from build123d import *

# Parameters (mm, degrees)
SKETCH_W        = 60
SKETCH_H        = 10
PAD_DEPTH       = 3
SKETCH001_R     = 2
POCKET_DEPTH    = 124.80412
SKETCH002_R     = 2.5
PAD001_DEPTH    = 40
FILLET_R        = 2
SKETCH003_W     = 12
SKETCH003_H     = 5
PAD002_DEPTH    = 5
SKETCH004_W     = 8
SKETCH004_H     = 3
POCKET001_DEPTH = 7.501
FILLET001_R     = 2
FILLET002_R     = 3


with BuildPart() as part:
    # Sketch → Pad (new body)
    with BuildSketch(Plane.XY):
        Rectangle(SKETCH_W, SKETCH_H)
    extrude(amount=PAD_DEPTH)

    # Sketch001 (on Face6 of Pad) → Pocket (cut, through all)
    with BuildSketch(Plane.XY.offset(3)):
        with Locations((-20, 0)):
            Circle(SKETCH001_R)
    pocket = extrude(amount=-POCKET_DEPTH, mode=Mode.SUBTRACT)

    # Mirrored: Pocket across Sketch001 V_Axis
    add(pocket.mirror(Plane(origin=(0, 0, 3), x_dir=(0, 0, 1), z_dir=(1, 0, 0))), mode=Mode.SUBTRACT)

    # Sketch002 (on Face5 of Mirrored) → Pad001 (join)
    with BuildSketch(Plane.XY.offset(3)):
        Circle(SKETCH002_R)
    extrude(amount=PAD001_DEPTH)

    # Fillet
    fillet_edges = [part.edges().sort_by_distance(p)[0] for p in [
        (-2.5, 0, 3),
    ]]
    fillet(fillet_edges, radius=FILLET_R)

    # Sketch003 (on Face11 of Fillet) → Pad002 (join)
    with BuildSketch(Plane.XY.offset(43)):
        Rectangle(SKETCH003_W, SKETCH003_H)
    extrude(amount=PAD002_DEPTH)

    # Sketch004 (on Face13 of Pad002) → Pocket001 (cut, through all)
    with BuildSketch(Plane.XZ.offset(2.5)):
        with Locations((0, 46.5)):
            Rectangle(SKETCH004_W, SKETCH004_H)
    extrude(amount=-POCKET001_DEPTH, mode=Mode.SUBTRACT)

    # Fillet001
    fillet001_edges = [part.edges().sort_by_distance(p)[0] for p in [
        (4, 0, 45),
        (-4, 0, 45),
    ]]
    fillet(fillet001_edges, radius=FILLET001_R)

    # Fillet002
    fillet002_edges = [part.edges().sort_by_distance(p)[0] for p in [
        (-6, 0, 43),
        (6, 0, 43),
    ]]
    fillet(fillet002_edges, radius=FILLET002_R)


solid = part.part
Can you work these out from the model? Positions are in its coordinate system, mm. A direction names the side the tool comes from. Coordinates: 2 decimals unless noted, no trailing zeros. Loops run counter-clockwise (first coordinate to the right, second up) from the corner with the lowest first, then second, coordinate; pieces in that order, holes last. Notation, with made-up numbers: M 46.5,49 L 90.5,49 A14 cw 90.5,67 Z; hole C -37.75,6 d3. An arc over 180 degrees is marked long. Return JSON: item names as keys, results as strings. Group by question number.
Item 1: Imagine slicing it at A-A (y = 0). Give the number of separate pieces and of enclosed holes in the cut face, and give its area (3 significant figures).
Item 2: If I drill on L1, parallel to Y at x = 20, z = 1; L2, parallel to Z at x = 25, y = 1; L3, parallel to X at y = -0.25, z = 28.5, over which ranges is the centre line in solid material (lowest first)? Write a range as from..to.
Item 3: Imagine slicing it at D-D (x = 19). Please give me the cut outline in (y, z).
Item 4: Imagine slicing it at B-B (x = -20). Please give me the cut outline in (y, z), and give its area (3 significant figures).
Item 5: I'm going to push flat-ended pins straight in: pin 1 Ø1 at (y, z) = (0.5, 25) entering from +X; pin 2 Ø3 at (x, y) = (-20, 0) entering from -Z; pin 3 Ø1.5 at (x, z) = (1, 45.5) entering from +Y; pin 4 Ø0.5 at (y, z) = (-0.5, 47.5) entering from -X. Where does each tip first touch, or does it pass through?
Item 6: Imagine slicing it at C-C (z = 24). Please give me the cut outline in (x, y), and give its area (3 significant figures).
Item 7: Thinking about a two-plate mould opening in Z: for faces 6 (the cylindrical face through (-5.1, 0.04, 43.86)), 7 (the cylindrical face through (-3.4, 0.04, 45.57)), 8 (the flat face through (0, 5, 1)), which applies, released by +Z, released by -Z, zero draft, split by the parting line, or undercut?
Item 8: On a 3-axis mill with a long thin cutter (end or side, diameter ignored), from which of +Z, -Z, +X, -X, +Y, -Y can I reach the whole of each face in a straight line? I mean faces 1 (the flat face through (6, 0, 47)), 2 (the flat face through (0, -2.5, 44)), 3 (the flat face through (-6, 0, 47)), 4 (the flat face through (0, 2.5, 44)), 5 (the cylindrical face through (5.14, 0.04, 43.9)). Say none if no direction works.
Verdict:
{
 "1": {"separate pieces": "3", "enclosed holes": "0", "area": "392 mm^2"},
 "2": {"L1": "y = -5..-2, 2..5", "L2": "z = 0..3", "L3": "x = -2.49..2.49"},
 "3": {"outline": "M -5,0 L -1.73,0 L -1.73,3 L -5,3 Z; M 1.73,0 L 5,0 L 5,3 L 1.73,3 Z"},
 "4": {"outline": "M -5,0 L -2,0 L -2,3 L -5,3 Z; M 2,0 L 5,0 L 5,3 L 2,3 Z", "area": "18.0 mm^2"},
 "5": {"pin 1": "stops at x = 2.5", "pin 2": "passes through", "pin 3": "stops at y = 2.5", "pin 4": "stops at x = -6"},
 "6": {"outline": "C 0,0 d5", "area": "19.6 mm^2"},
 "7": {"face 6": "undercut", "face 7": "released by +Z", "face 8": "zero draft"},
 "8": {"face 1": "+Z, +X, +Y, -Y", "face 2": "+Z, +X, -X, -Y", "face 3": "+Z, -X, +Y, -Y", "face 4": "+Z, +X, -X, +Y", "face 5": "+X, +Y, -Y"}
}
